Autodesk Inventor part; units mm, degrees
ref_plane "YZ Plane" through (0, 0, 0) normal (1, 0, 0) x (0, 1, 0)
ref_plane "XZ Plane" through (0, 0, 0) normal (0, 1, 0) x (-1, 0, 0)
ref_plane "XY Plane" through (0, 0, 0) normal (0, 0, 1) x (1, 0, 0)
sketch "Sketch1" plane through (0, 0, 0) normal (0, 0, 1) x (1, 0, 0)
  line L0 (0, 0) -> (0, 20)
  circle A0 centre (6.5, 20) radius 6.5
  circle A1 centre (6.5, 20) radius 4
  line L1 (13, 20) -> (13, 0)
  line L2 (13, 0) -> (0, 0)
  dimension "d0" = 20
extrude "Extrusion1" add sketch "Sketch1" along normal mid plane 49
sketch "Sketch2" plane through (13, 0, 24.5) normal (1, 0, 0) x (0, 0, -1)
  line L0 (49, 0) -> (0, 0)
  line L1 (0, 0) -> (0, -40)
  line L2 (0, -40) -> (49, -40)
  line L3 (49, -40) -> (49, 0)
  line L4 (0, -40) -> (24.5, -40)
  line L5 (24.5, -40) -> (24.5, -20)
  circle A0 centre (24.5, -20) radius 20
  circle A1 centre (24.5, -20) radius 16.85
  point P0 (24.5, 0)
  dimension "d11" = 40
  dimension "d12" = 24.5
  dimension "d13" = 20
  dimension "d14" = 33.7
extrude "Extrusion2" add sketch "Sketch2" along normal mid plane 50
fillet "Fillet1" radius 5 1 edges at (13, 0, 0)
fillet "Fillet2" radius 5 1 edges at (0, 0, 0)
properties part number "PlacaExcavacion2"
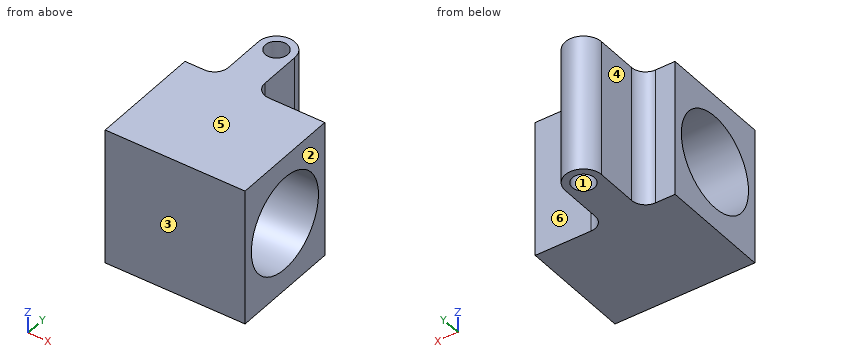
Check sheet for the modelled part. Datum: model origin and axes. Units: mm. Face numbers are marked on the shaded views. A direction names the side the tool comes from. Give positions to 0.01 mm unless a question says otherwise; leave off trailing zeros. Loops run counter-clockwise (first coordinate to the right, second up) from the corner with the lowest first, then second, coordinate; pieces in that order, holes last. Notation, with made-up numbers: (14, -38) - (37, -38) arc R19 ccw to (37, -24) - close; hole circle Ø1 at (-7.75, 46.5). An arc over 180 degrees is marked (long way). One line per question, with ' | ' between items. Start each with the question number.
1. Cross-section at A-A, the plane z = 0. Enter the section's corners in (x, y), plus the area to 3 significant figures.
2. Cross-section at B-B, the plane y = -20. Enter the section's corners in (x, z), plus the area to 3 significant figures.
3. Cross-section at D-D, the plane z = 18.5. Enter the section's corners in (x, y).
4. Cross-section at C-C, the plane x = 28. Enter the section's corners in (y, z).
5. Material ranges on line 1 along Y through (x, z) = (6, -11); line 2 along Y through (x, z) = (6.5, 0); line 3 along Y through (x, z) = (20.5, 0), recorded low to high. Write a range as [from, to].
6. Set-up check for the marked faces 4, 5 and 6: record each of +Z, -Z, +X, -X, +Y, -Y from which the full face is reachable in a straight line by a thin tool's end or side.
7. Draft check along X on the marked faces 1, 2 and 3. Enter one of: released by +X, released by -X, zero draft, split by the parting line, or undercut.
8. Gauge pin test, flat ends, axial feed: pin 1 Ø10 at (x, z) = (29.5, 9) entering from +Y; pin 2 Ø16.5 at (y, z) = (9.5, -11.5) entering from +X; pin 3 Ø12 at (y, z) = (13.5, 10.5) entering from -X. Record the tip position at first contact, or that the pin passes through.
Check result:
1) outline: (-12, -40) - (38, -40) - (38, -36.85) - (-12, -36.85) - close; (-12, -3.15) - (38, -3.15) - (38, 0) - (18, 0) arc R5 cw to (13, 5) - (13, 20) arc R6.5 ccw to (0, 20) - (0, 5) arc R5 cw to (-5, 0) - (-12, 0) - close; hole circle Ø8 at (6.5, 20) | area: 602 mm2
2) outline: (-12, -24.5) - (38, -24.5) - (38, -16.85) - (-12, -16.85) - close; (-12, 16.85) - (38, 16.85) - (38, 24.5) - (-12, 24.5) - close | area: 765 mm2
3) outline: (-12, -40) - (38, -40) - (38, 0) - (18, 0) arc R5 cw to (13, 5) - (13, 20) arc R6.5 ccw to (0, 20) - (0, 5) arc R5 cw to (-5, 0) - (-12, 0) - close; hole circle Ø8 at (6.5, 20)
4) outline: (-40, -24.5) - (0, -24.5) - (0, 24.5) - (-40, 24.5) - close; hole circle Ø33.7 at (-20, 0)
5) line 1: y = [-40, -32.76], [-7.24, 16.03], [23.97, 26.48] | line 2: y = [-40, -36.85], [-3.15, 16], [24, 26.5] | line 3: y = [-40, -36.85], [-3.15, 0]
6) face 4: +Z, -Z, -X, +Y | face 5: +Z, +X, -X, +Y, -Y | face 6: +Z, -Z, +X, +Y
7) face 1: undercut | face 2: released by +X | face 3: zero draft
8) pin 1: stops at y = 0 | pin 2: stops at x = 14.69 | pin 3: stops at x = 0
